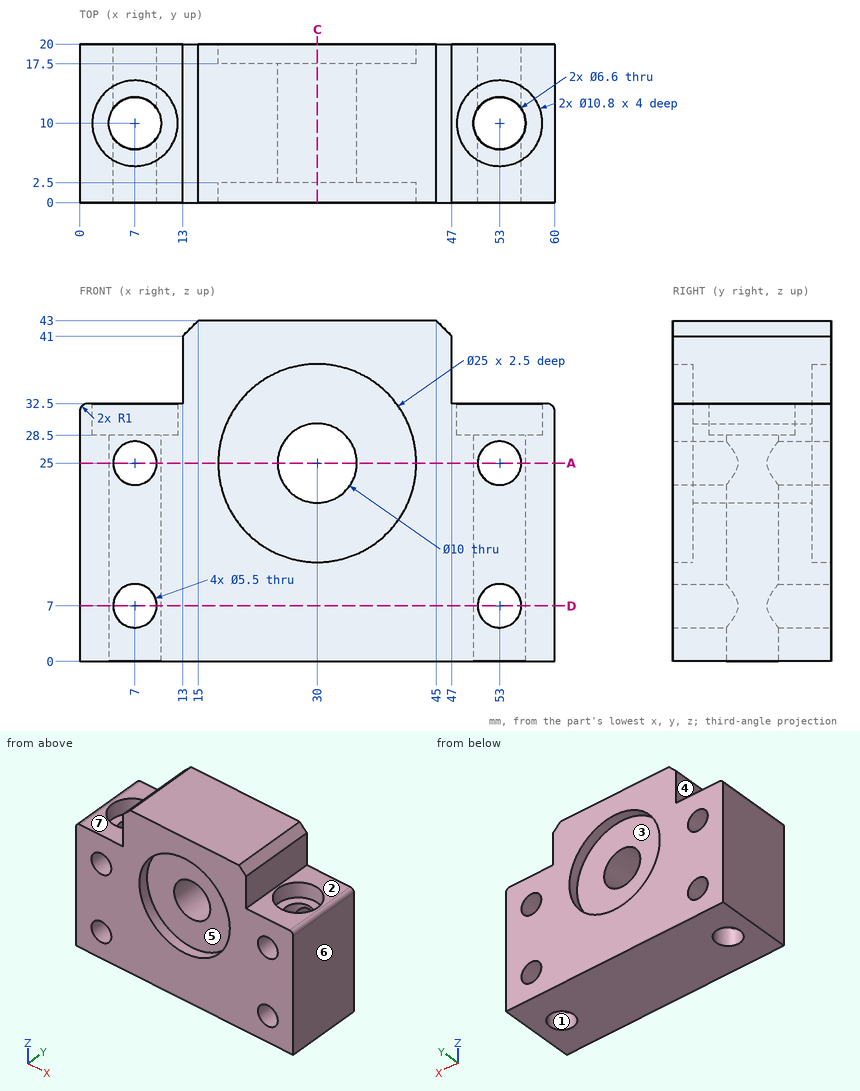
Verification items for this drawing (mm, ordinates from the low corner). A direction names the side the tool comes from. Coordinates: 2 decimals unless noted, no trailing zeros. Write each loop counter-clockwise with the first axis right and the second up, starting at its lowest first coordinate (ties: lowest second). Pieces come first, ordered by that corner, then holes. Notation, with made-up numbers: (84, 40) - (89, 40) arc R32 ccw to (89, 76) - close; hole circle Ø1 at (-32.5, -15). An arc over 180 degrees is marked (long way). One line per question, with ' | ' between items.
Item 1: Mould release check, pull along X, two halves, no side actions. Record for the marked faces 5, 6 and 7: pulls with the +X half, pulls with the -X half, needs draft (parallel to the pull), parting line crosses it, or undercut.
Determined:
face 5: undercut | face 6: pulls with the +X half | face 7: needs draft
Item 2: Thickness scan on line 1 (Z direction, x = 7, y = 3.5); line 2 (Z direction, x = 30, y = 19.4); line 3 (Y direction, x = 53, z = 30). Record the ranges inside material, lowest first. Write a range as [from, to].
Determined:
line 1: z = [0, 4.25], [9.75, 22.25], [27.75, 32.5] | line 2: z = [0, 12.5], [37.5, 43] | line 3: y = [0, 4.6], [15.4, 20]
Item 3: Sectioned sample at C-C on x = 30. Record the boundary of the cut face in (y, z), plus the area to 3 significant figures.
Determined:
outline: (0, 0) - (20, 0) - (20, 12.5) - (17.5, 12.5) - (17.5, 20) - (2.5, 20) - (2.5, 12.5) - (0, 12.5) - close; (0, 37.5) - (2.5, 37.5) - (2.5, 30) - (17.5, 30) - (17.5, 37.5) - (20, 37.5) - (20, 43) - (0, 43) - close | area: 585 mm2
Item 4: Sectioned sample at A-A on z = 25. Give the number of separate pieces and of enclosed holes in the cut face, plus the area to 3 significant figures.
Determined:
separate pieces: 4 | enclosed holes: 0 | area: 700 mm2
Item 5: Access from +Z, -Z, +X, -X, +Y, -Y to the whole of each face (thin tool, end or side, straight path). Record for the marked faces 1, 2, 3 and 4.
Determined:
face 1: +Z, -Z | face 2: +Z, +X, +Y, -Y | face 3: +Y | face 4: +Z, -X, +Y, -Y
Item 6: Sectioned sample at D-D on z = 7. Record the boundary of the cut face in (x, y), plus the area to 3 significant figures.
Determined:
outline: (0, 0) - (4.25, 0) - (4.25, 8.18) arc R3.3 cw to (4.25, 11.82) - (4.25, 20) - (0, 20) - close; (9.75, 0) - (50.25, 0) - (50.25, 8.18) arc R3.3 cw to (50.25, 11.82) - (50.25, 20) - (9.75, 20) - (9.75, 11.82) arc R3.3 cw to (9.75, 8.18) - close; (55.75, 0) - (60, 0) - (60, 20) - (55.75, 20) - (55.75, 11.82) arc R3.3 cw to (55.75, 8.18) - close | area: 975 mm2
Item 7: Gauge pin test, flat ends, axial feed: P1, Ø5.5, axis at x = 53.5, y = 9, coming from the +Z side; P2, Ø3, axis at y = 16, z = 14.5, coming from the -X side; P3, Ø16, axis at x = 30, z = 25, coming from the -Y side; P4, Ø3.5, axis at x = 7, z = 25, coming from the +Y side. Record the tip position at first contact, or that the pin passes through.
Determined:
P1: stops at z = 28.5 | P2: stops at x = 0 | P3: stops at y = 2.5 | P4: passes through
